Input: part model. Units: mm. Frame: model coordinates. Coordinates: 2 decimals unless noted, no trailing zeros. Loops run counter-clockwise (first coordinate to the right, second up) from the corner with the lowest first, then second, coordinate; pieces in that order, holes last. Notation, with made-up numbers: (26, 15.5) - (53, 15.5) arc R31 cw to (53, 40.5) - close; hole circle Ø6 at (8.5, 75). An arc over 180 degrees is marked (long way). Use a Markdown table: item, result. Add a question column.
1. Draft query along X for faces 1 (the face through (34, 1, -10)), 2 (the face through (5.306, 1.331, -2.735)), 3 (the face through (17, 2.7, -10)). Return one class per face: released by +X, released by -X, zero draft, split by the parting line, or undercut.
2. Section query B-B on x = 4.5. Return the cut outline in (y, z), then the cut area to 3 significant figures.
3. Section query C-C on y = 0.75. Return the cut outline in (x, z).
4. Ray query, L1, parallel to Z at x = 4.5, y = 2; L2, parallel to Z at x = 4, y = 2.3; L3, parallel to X at y = 0.95, z = -3. Return the intervals inside material, ascending. Write a range as [from, to].
5. Contact query for flat-ended pins moving along their axis: P1, Ø3, axis at x = 13.5, z = -2.5, coming from the -Y side; P2, Ø1.8, axis at x = 4.5, z = -17, coming from the +Y side. Output: stop coordinate, or through.
6. Section query A-A on z = -17. Return the cut outline in (x, y).
Autodesk Inventor part; units mm, degrees
ref_plane "YZ Plane" through (0, 0, 0) normal (1, 0, 0) x (0, 1, 0)
ref_plane "XZ Plane" through (0, 0, 0) normal (0, 1, 0) x (-1, 0, 0)
ref_plane "XY Plane" through (0, 0, 0) normal (0, 0, 1) x (1, 0, 0)
sketch "Sketch1" plane through (0, 0, 0) normal (0, 1, 0) x (-1, 0, 0)
  line L0 (0, 0) -> (-34, 0)
  line L1 (-34, 0) -> (-34, -21)
  line L2 (-34, -21) -> (0, -21)
  line L3 (0, -21) -> (0, 0)
  dimension "d0" = 34
  dimension "d1" = 21
extrude "Extrusion1" add sketch "Sketch1" along normal blind 2.7
sketch "Sketch2" plane through (0, 0, 0) normal (0, -1, 0) x (1, 0, 0)
  line L0 (0, 0) -> (4.5, 0)
  line L1 (0, 0) -> (34, 0)
  circle A0 centre (4.5, -4) radius 1.5
  line L2 (34, 0) -> (34, -21)
  line L3 (0, -21) -> (0, 0)
  circle A1 centre (4.5, -17) radius 1.5
  dimension "d4" = 4.5
  dimension "d6" = 3
extrude "Extrusion2" cut sketch "Sketch2" against normal blind 2.7
properties part number "Scheda cella di carico"
Resolved:
| question | item | result |
|---|---|---|
| 1 | face 1 | released by +X |
| 1 | face 2 | undercut |
| 1 | face 3 | zero draft |
| 2 | outline | (0, -21) - (2.7, -21) - (2.7, -18.5) - (0, -18.5) - close; (0, -15.5) - (2.7, -15.5) - (2.7, -5.5) - (0, -5.5) - close; (0, -2.5) - (2.7, -2.5) - (2.7, 0) - (0, 0) - close |
| 2 | area | 40.5 mm² |
| 3 | outline | (0, -21) - (34, -21) - (34, 0) - (0, 0) - close; hole circle Ø3 at (4.5, -17); hole circle Ø3 at (4.5, -4) |
| 4 | L1 | [-21, -18.5], [-15.5, -5.5], [-2.5, 0] |
| 4 | L2 | [-21, -18.41], [-15.59, -5.41], [-2.59, 0] |
| 4 | L3 | [0, 3.38], [5.62, 34] |
| 5 | P1 | y = 0 |
| 5 | P2 | through |
| 6 | outline | (0, 0) - (3, 0) - (3, 2.7) - (0, 2.7) - close; (6, 0) - (34, 0) - (34, 2.7) - (6, 2.7) - close |
